Read the model definition and answer for the solid it produces. Units are mm, in the model's axes. A direction names the side the tool comes from. Give positions to 0.01 mm unless a question says otherwise; leave off trailing zeros. Write item = value, one per line.
```python
from build123d import *


with BuildPart() as part:
    # Esquisse1 → Base-Révolution (revolve)
    with BuildSketch(Plane(origin=(0, 0, 0), x_dir=(1, 0, 0), z_dir=(0, 1, 0)), mode=Mode.PRIVATE) as base_r_volution_sk:
        with BuildLine():
            Line((0, 15.683012702), (0, 17.166666667))
            ThreePointArc((0, 17.166666667), (0.097631073, 17.402368927), (0.333333333, 17.5))
            Line((0.333333333, 17.5), (4.666666667, 17.5))
            ThreePointArc((4.666666667, 17.5), (4.902368927, 17.402368927), (5, 17.166666667))
            Line((5, 17.166666667), (5, 16.75))
            Line((5, 16.75), (4.666666667, 16.75))
            Line((4.666666667, 16.75), (4.666666667, 17.25))
            Line((4.666666667, 17.25), (4.166666667, 17.25))
            Line((4.166666667, 17.25), (4.166666667, 17))
            Line((4.166666667, 17), (0.5, 17))
            Line((0.5, 17), (0.5, 15.816987298))
            Line((0.5, 15.816987298), (0.971687836, 15))
            Line((0.971687836, 15), (2.625, 15))
            ThreePointArc((2.625, 15), (2.936586758, 15.36959946), (3.353553391, 15.125))
            Line((3.353553391, 15.125), (3.75, 15.125))
            Line((3.75, 15.125), (3.75, 14.75))
            Line((3.75, 14.75), (3, 14))
            Line((3, 14), (1.62626129, 14.5))
            Line((1.62626129, 14.5), (1.293589427, 14.5))
            Line((1.293589427, 14.5), (0.427564023, 14))
            Line((0.427564023, 14), (0.25, 14.30754991))
            Line((0.25, 14.30754991), (0.583333333, 14.5))
            Line((0.583333333, 14.5), (0.333333333, 14.5))
            ThreePointArc((0.333333333, 14.5), (0.097631073, 14.597631073), (0, 14.833333333))
            Line((0, 14.833333333), (0, 15.25))
            Line((0, 15.25), (0.25, 15.25))
            Line((0.25, 15.25), (0, 15.683012702))
        make_face()
    revolve(base_r_volution_sk.sketch.rotate(Axis((0, 0, 0), (1, 0, 0)), 180), axis=Axis((0, 0, 0), (1, 0, 0)))


solid = part.part
```
1) Find the intervals of material crossed by probe 1 along Y at (x, z) = (2.7, -6); probe 2 along Y at (x, z) = (2.1, -8.5); probe 3 along Y at (x, z) = (4.45, 0), in increasing order.
Output:
probe_1 = -16.44 to -15.91, -13.99 to -12.77, 12.77 to 13.99, 15.91 to 16.44
probe_2 = -15.3 to -14.72, -12.36 to -11.53, 11.53 to 12.36, 14.72 to 15.3
probe_3 = -17.5 to -17.25, 17.25 to 17.5
2) Each of these flat-tipped pins is pushed along its axis until it touches: P1, Ø10, axis at y = -5, z = 13.5, coming from the -X side; P2, Ø1, axis at x = 3, y = -2, coming from the +Z side; P3, Ø1.5, axis at x = 0.5, z = -4.5, coming from the -Y side; P4, Ø1.5, axis at x = 1, z = -10.5, coming from the -Y side. Where does it stop, or does it pass through?
Output:
P1 = 0
P2 = 17.44
P3 = -17.09
P4 = -14.53
3) The mould has two halves that part along Z. Classify faces 1 (the face through (0, 14, -8)), 2 (the face through (4.667, -16.7, 2.6)), 3 (the face through (2.53, 17.084, -3.794)): pulls with the +Z half, pulls with the -Z half, needs draft (parallel to the pull), parting line crosses it, or undercut.
Output:
face_1 = needs draft
face_2 = undercut
face_3 = parting line crosses it
4) A tool of negligible diameter and unlimited length cuts with its end or side. For faces 4 (the face through (0.5, 11.3, 11.3)), 5 (the face through (3.75, 6.65, 13.37)), 6 (the face through (0, 14.614, -3.318)), from which of +Z, -Z, +X, -X, +Y, -Y can it reach the whole face along a straight path? Write none if from no direction.
Output:
face_4 = none
face_5 = +X
face_6 = +Z, -Z, -X, +Y, -Y
